Could you check a few things on this model? Use its own coordinates, in mm. Face numbers are marked on the shaded views. A direction names the side the tool comes from. Coordinates: 2 decimals unless noted, no trailing zeros. Write each loop counter-clockwise with the first axis right and the second up, starting at its lowest first coordinate (ties: lowest second). Pieces come first, ordered by that corner, then holes. Notation, with made-up numbers: (-26, 26.25) - (28, 26.25) arc R23 ccw to (28, 63.25) - close; hole circle Ø10 at (65.25, 6). An arc over 180 degrees is marked (long way). Write item = value, one per line. Start each with the question number.
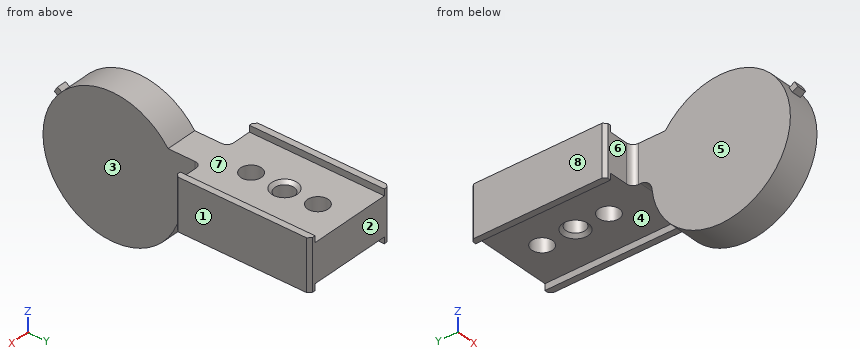
Autodesk Inventor part; units mm, degrees
ref_plane "GRIFF_XY" through (0, 0, 0) normal (1, 0, 0) x (0, 0, -1)
ref_plane "GRIFF_YZ" through (0, 0, 0) normal (0, 0, -1) x (0, 1, 0)
ref_plane "GRIFF_ZX" through (0, 0, 0) normal (0, 1, 0) x (1, 0, 0)
sketch "Sketch_1" plane through (0, 0, 0) normal (1, 0, 0) x (0, 1, 0)
  arc A0 (8.7499, 6.5) -> (10.8427, -1.1157) centre (0, 0) ccw
  arc A1 (12.6333, 0.5) -> (10.8427, -1.1157) centre (12.6333, -1.3) ccw
  line L0 (12.6333, 0.5) -> (35.2, 0.5)
  line L1 (35.2, 0.5) -> (35.2, 6.5)
  line L2 (35.2, 6.5) -> (8.7499, 6.5)
extrude "Extrusion1" add sketch "Sketch_1" along normal mid plane 13
sketch "Sketch_2" plane through (0, 0, 0) normal (0, 0, 1) x (1, 0, 0)
  line L0 (-6.5, -21.8) -> (6.5, -21.8)
  line L1 (6.5, -21.8) -> (6.5, 14)
  line L2 (6.5, 14) -> (3.5, 14)
  arc A0 (3.5, 14) -> (2.5, 13) centre (3.5, 13) ccw
  line L3 (2.5, 13) -> (2.5, -18.8)
  line L4 (2.5, -18.8) -> (-2.5, -18.8)
  line L5 (-2.5, -18.8) -> (-2.5, 13)
  arc A1 (-2.5, 13) -> (-3.5, 14) centre (-3.5, 13) ccw
  line L6 (-3.5, 14) -> (-6.5, 14)
  line L7 (-6.5, 14) -> (-6.5, -21.8)
extrude "Extrusion2" cut sketch "Sketch_2" along normal mid plane 30
sketch "Sketch_3" plane through (0, 0, 7.5) normal (0, 0, 1) x (1, 0, 0)
  line L0 (6.5, 14) -> (7, 14)
  line L1 (7, 14) -> (7.5, 14.5)
  line L2 (7.5, 14.5) -> (7.5, 34.7)
  line L3 (7.5, 34.7) -> (7, 35.2)
  line L4 (7, 35.2) -> (6.5, 35.2)
  line L5 (6.5, 35.2) -> (6.5, 14)
extrude "Extrusion3" add sketch "Sketch_3" against normal blind 8
sketch "Sketch_4" plane through (0, 0, 7.5) normal (0, 0, 1) x (1, 0, 0)
  line L0 (-7.5, 14.5) -> (-7, 14)
  line L1 (-7, 14) -> (-6.5, 14)
  line L2 (-6.5, 14) -> (-6.5, 35.2)
  line L3 (-6.5, 35.2) -> (-7, 35.2)
  line L4 (-7, 35.2) -> (-7.5, 34.7)
  line L5 (-7.5, 34.7) -> (-7.5, 14.5)
extrude "Extrusion4" add sketch "Sketch_4" against normal blind 8
sketch "Sketch_5" plane through (0, 0, 0) normal (1, 0, 0) x (0, 1, 0)
  line L0 (24.95, 0.5) -> (24.95, 6.5)
  line L1 (24.95, 6.5) -> (26.95, 6.5)
  line L2 (26.95, 6.5) -> (26.45, 6)
  line L3 (26.45, 6) -> (26.45, 1)
  line L4 (26.45, 1) -> (26.95, 0.5)
  line L5 (26.95, 0.5) -> (24.95, 0.5)
  line L6 (24.95, 0.5) -> (24.95, 6.5)
revolve "Revolution1" cut sketch "Sketch_5" angle 360 about axis through (0, 24.95, 0.5) along (0, 0, -1)
sketch "Sketch6" plane through (-2.5, 8.7499, 6.5) normal (0, 0, 1) x (1, 0, 0)
  point P0 (2.5, 10.9501)
hole "Hole1" at (0, 19.7, 6.5) direction (0, 0, -1) diameter 3.242 depth 6
sketch "Sketch7" plane through (-2.5, 8.7499, 6.5) normal (0, 0, 1) x (1, 0, 0)
  point P0 (2.5, 21.4501)
hole "Hole2" at (0, 30.2, 6.5) direction (0, 0, -1) diameter 3.242 depth 6
sketch "Sketch_9" plane through (0, 0, 0) normal (1, 0, 0) x (0, 1, 0)
  arc A0 (-10.0918, 6.306) -> (-10.603, 5.4025) centre (0, 0) ccw
  line L0 (-10.603, 5.4025) -> (0, 0)
  line L1 (0, 0) -> (-10.0918, 6.306)
extrude "Extrusion5" add sketch "Sketch_9" along normal mid plane 1.5
ref_plane "GRIFF_XY" through (0, 0, 0) normal (1, 0, 0) x (0, 0, -1)
ref_plane "GRIFF_YZ" through (0, 0, 0) normal (0, 0, -1) x (0, 1, 0)
ref_plane "GRIFF_ZX" through (0, 0, 0) normal (0, 1, 0) x (1, 0, 0)
properties part number "1310162 DHRS-25-A---(Griff)"
1) Suppose I cut it at D-D on z = 3.75. Please give me the cut outline in (x, y), plus the area to 3 significant figures.
2) If I drill on probe 1 along X at (y, z) = (19.7, 1.85); probe 2 along X at (y, z) = (22.5, 0.25); probe 3 along Z at (x, y) = (-6, 21.5), over which ranges is the centre line in solid material (lowest first)? Write a range as [from, to].
3) Thinking about a two-plate mould opening in X: for the marked faces 6, 7 and 8, which applies, +X half, -X half, draft (parallel to the pull), parting line (faces both ways), or undercut?
4) Suppose I cut it at C-C on y = 28. Please give me the cut outline in (x, z), plus the area to 3 significant figures.
5) For P1, Ø11, axis at y = -4, z = -5.5, coming from the +X side; P2, Ø2.5, axis at x = 0, y = 24.95, coming from the -Z side; P3, Ø1.1, axis at x = 7, y = 27, coming from the +Z side; P4, Ø0.7, axis at y = -10, z = 5.5, coming from the -X side, each with a flat end and sliding along its axis, tell me the tip position at first contact or that it passes through.
6) Suppose I cut it at A-A on x = 0. Please give me the cut outline in (y, z).
7) Which directions (+Z, -Z, +X, -X, +Y, -Y) give clear straight access to the entire face, cutting with the end or side of a thin tool? Please do the marked faces 1, 2, 3, 4 and 5.
8) Suppose I cut it at B-B on y = 19.7. Please give me the cut outline in (x, z), plus the area to 3 significant figures.
Reply:
q1.outline = (-7.5, 14.5) - (-7, 14) - (-3.5, 14) arc R1 cw to (-2.5, 13) - (-2.5, -10.23) - (2.5, -10.23) - (2.5, 13) arc R1 cw to (3.5, 14) - (7, 14) - (7.5, 14.5) - (7.5, 34.7) - (7, 35.2) - (-7, 35.2) - (-7.5, 34.7) - close; hole circle Ø3.24 at (0, 19.7); hole circle Ø3.24 at (0, 30.2); hole circle Ø3 at (0, 24.95)
q1.area = 416 mm^2
q2.probe_1 = [-7.5, -1.62], [1.62, 7.5]
q2.probe_2 = [-7.5, -6.5], [6.5, 7.5]
q2.probe_3 = [0.5, 6.5]
q3.face_6 = draft
q3.face_7 = undercut
q3.face_8 = -X half
q4.outline = (-7.5, -0.5) - (-6.5, -0.5) - (-6.5, 0.5) - (6.5, 0.5) - (6.5, -0.5) - (7.5, -0.5) - (7.5, 7.5) - (6.5, 7.5) - (6.5, 6.5) - (-6.5, 6.5) - (-6.5, 7.5) - (-7.5, 7.5) - close
q4.area = 94.0 mm^2
q5.P1 = 2.5
q5.P2 = through
q5.P3 = 7.5
q5.P4 = -0.75
q6.outline = (-10.6, 5.4) - (-9.71, 4.95) arc R10.9 ccw (long way) to (10.84, -1.12) arc R1.8 cw to (12.63, 0.5) - (18.08, 0.5) - (18.08, 6.5) - (8.75, 6.5) arc R10.9 ccw to (-9.24, 5.78) - (-10.09, 6.31) arc R11.91 ccw to start; (21.32, 0.5) - (22.95, 0.5) - (23.45, 1) - (23.45, 6) - (22.95, 6.5) - (21.32, 6.5) - close; (26.45, 1) - (26.95, 0.5) - (28.58, 0.5) - (28.58, 6.5) - (26.95, 6.5) - (26.45, 6) - close; (31.82, 0.5) - (35.2, 0.5) - (35.2, 6.5) - (31.82, 6.5) - close
q7.face_1 = +Z, -Z, +X, +Y, -Y
q7.face_2 = +Z, -Z, +X, -X, +Y
q7.face_3 = +Z, -Z, +X, -Y
q7.face_4 = -Z, +Y
q7.face_5 = +Z, -Z, -X, -Y
q8.outline = (-7.5, -0.5) - (-6.5, -0.5) - (-6.5, 0.5) - (-1.62, 0.5) - (-1.62, 6.5) - (-6.5, 6.5) - (-6.5, 7.5) - (-7.5, 7.5) - close; (1.62, 0.5) - (6.5, 0.5) - (6.5, -0.5) - (7.5, -0.5) - (7.5, 7.5) - (6.5, 7.5) - (6.5, 6.5) - (1.62, 6.5) - close
q8.area = 74.5 mm^2
